Can you work these out from the model? Positions are in its coordinate system, mm. A direction names the side the tool comes from. Coordinates: 2 decimals unless noted, no trailing zeros. Order: outer loops, then holes, each group sorted by start corner. A loop starts at its lowest first (then second) coordinate and runs counter-clockwise, first axis right, second up. Notation, with made-up numbers: (-32.75, 77.5) -> (-13.75, 77.5) arc R29 cw to (-13.75, 106.5) -> close; hole circle Ø4 at (8, 28). An arc over 180 degrees is marked (long way). Answer in a Markdown table with one row per item.
```python
from build123d import *

# Parameters (mm, degrees)
F3_W        = 10
F3_H        = 25.1
F4_DEPTH    = 29.1
F5_DEPTH    = 27.1
F6_DEPTH    = 2
F7_T1_DEPTH = 52.9484800354


# Not quite as in the source:
# - a fillet or chamfer that OpenCascade refuses, or shapes differently, is made with other operations: its cross-section is extruded or revolved along the edge and cut away or added


with BuildPart() as f4:
    # F3 (on Top) → F4 (new body)
    with BuildSketch(Plane.XY):
        Rectangle(F3_W, F3_H)
        with BuildLine():
            Line((5, -12.55), (-5, -12.55))
            Line((-5, -12.55), (-5, -22.55))
            Line((-5, -22.55), (-1.5, -22.55))
            Line((-1.5, -22.55), (-1.5, -20.1480762114))
            ThreePointArc((-1.5, -20.1480762114), (0, -14.55), (1.5, -20.1480762114))
            Line((1.5, -20.1480762114), (1.5, -22.55))
            Line((1.5, -22.55), (5, -22.55))
            Line((5, -22.55), (5, -12.55))
        make_face()
    extrude(amount=F4_DEPTH)

    # F3 (on Top) → F5 (cut)
    with BuildSketch(Plane.XY):
        Rectangle(F3_W, F3_H)
    extrude(amount=F5_DEPTH, mode=Mode.SUBTRACT)

    # F3 (on Top) → F6 (join)
    with BuildSketch(Plane.XY):
        Rectangle(F3_W, F3_H)
        with BuildLine():
            Line((5, -12.55), (-5, -12.55))
            Line((-5, -12.55), (-5, -22.55))
            Line((-5, -22.55), (-1.5, -22.55))
            Line((-1.5, -22.55), (-1.5, -20.1480762114))
            ThreePointArc((-1.5, -20.1480762114), (0, -14.55), (1.5, -20.1480762114))
            Line((1.5, -20.1480762114), (1.5, -22.55))
            Line((1.5, -22.55), (5, -22.55))
            Line((5, -22.55), (5, -12.55))
        make_face()
    extrude(amount=F6_DEPTH)

    # F7: fillet of radius 5 on 2 edges, made by hand

    # F7_s2 → F7_t1 (cut)
    with BuildSketch(Plane.XY.offset(-11.9242400177)):
        with BuildLine():
            ThreePointArc((-1.5, -22.55), (-4.0311288741, -20.7383438845), (-5, -17.7803039929))
            Line((-5, -17.7803039929), (-5, -22.55))
            Line((-5, -22.55), (-1.5, -22.55))
        make_face()
        with BuildLine():
            ThreePointArc((5, -17.7803039929), (4.0311288741, -20.7383438845), (1.5, -22.55))
            Line((1.5, -22.55), (5, -22.55))
            Line((5, -22.55), (5, -17.7803039929))
        make_face()
    extrude(amount=F7_T1_DEPTH, mode=Mode.SUBTRACT)


solid = f4.part
```
(1) Suppose I cut it at B-B (x = 0). Please give me the cut outline in (y, z), and give its area (3 significant figures).
Response values:
| item | result |
|---|---|
| outline | (-14.55, 0) -> (12.55, 0) -> (12.55, 2) -> (-12.55, 2) -> (-12.55, 27.1) -> (12.55, 27.1) -> (12.55, 29.1) -> (-14.55, 29.1) -> close |
| area | 159 mm2 |
(2) I need wall thicknesses on line 1 (X direction, y = -17.55, z = 11); line 2 (Z direction, x = 2.5, y = 3.5); line 3 (Y direction, x = 0, z = 6.25). Which ranges of each line are inside material? Lowest first, please. Write a range as [from, to].
Response values:
| item | result |
|---|---|
| line 1 | [-5, -3], [3, 5] |
| line 2 | [0, 2], [27.1, 29.1] |
| line 3 | [-14.55, -12.55] |
(3) Suppose I cut it at A-A (y = 2.5). Please give me the cut outline in (x, z), and give its area (3 significant figures).
Response values:
| item | result |
|---|---|
| outline | (-5, 0) -> (5, 0) -> (5, 2) -> (-5, 2) -> close; (-5, 27.1) -> (5, 27.1) -> (5, 29.1) -> (-5, 29.1) -> close |
| area | 40.0 mm2 |
(4) Suppose I cut it at C-C (z = 11.5). Please give me the cut outline in (x, y), and give its area (3 significant figures).
Response values:
| item | result |
|---|---|
| outline | (-5, -17.78) arc R5 ccw to (-1.5, -22.55) -> (-1.5, -20.15) arc R3 cw (long way) to (1.5, -20.15) -> (1.5, -22.55) arc R5 ccw to (5, -17.78) -> (5, -12.55) -> (-5, -12.55) -> close |
| area | 56.4 mm2 |
(5) We'd pull the mould along X, two halves only. Please class faces 1 (the flat face through (0, -5, 29.1)), 2 (the cylindrical face through (-0.11, -14.552, 14.346)), 3 (the flat face through (1.5, -21, 14)), 4 (the cylindrical face through (-4.005, -20.774, 14.346)): +X half, -X half, draft (parallel to the pull), parting line (faces both ways), or undercut.
Response values:
| item | result |
|---|---|
| face 1 | draft |
| face 2 | undercut |
| face 3 | undercut |
| face 4 | -X half |
(6) On a 3-axis mill with a long thin cutter (end or side, diameter ignored), from which of +Z, -Z, +X, -X, +Y, -Y can I reach the whole of each face in a straight line? I mean faces 5 (the flat face through (0, 0, 2)), 6 (the flat face through (-1.5, -21, 14)), 7 (the flat face through (0, 12.55, 28)). Say none if no direction works.
Response values:
| item | result |
|---|---|
| face 5 | +X, -X, +Y |
| face 6 | +Z, -Z, -Y |
| face 7 | +Z, -Z, +X, -X, +Y |
(7) Will these pins go through, and if not, where does the flat tip stop? pin 1 Ø4 at (x, z) = (0, 13.5) entering from -Y; pin 2 Ø2.5 at (y, z) = (-21.5, 8) entering from +X; pin 3 Ø0.7 at (y, z) = (-21, 10) entering from -X; pin 4 Ø3 at (x, z) = (2.5, 25) entering from +Y.
Response values:
| item | result |
|---|---|
| pin 1 | y = -22.55 |
| pin 2 | x = 4.35 |
| pin 3 | x = -4.09 |
| pin 4 | y = -12.55 |
